```python
from build123d import *

# Parameters (mm, degrees)
F0_W     = 76.350024
F0_H     = 76.350024
F0_R     = 2.15265
F0_R_2   = 3
F0_R_3   = 15.497899
F1_DEPTH = 5.08
F2_R     = 4.7625


with BuildPart() as f1:
    # F0 (on Top) → F1 (new body)
    with BuildSketch(Plane.XY):
        Rectangle(F0_W, F0_H)
        with Locations((-33.412512, -33.412512)):
            Circle(F0_R, mode=Mode.SUBTRACT)
        with Locations((0, -32.000012)):
            Circle(F0_R_2, mode=Mode.SUBTRACT)
        with Locations((33.412512, -33.412512)):
            Circle(F0_R, mode=Mode.SUBTRACT)
        with Locations((-27.712823, 16.000006)):
            Circle(F0_R_2, mode=Mode.SUBTRACT)
        with Locations((-33.412512, 33.412512)):
            Circle(F0_R, mode=Mode.SUBTRACT)
        Circle(F0_R_3, mode=Mode.SUBTRACT)
        with Locations((27.712823, 16.000006)):
            Circle(F0_R_2, mode=Mode.SUBTRACT)
        with Locations((33.412512, 33.412512)):
            Circle(F0_R, mode=Mode.SUBTRACT)
    extrude(amount=F1_DEPTH)

    # F2
    f2_edges = [f1.edges().sort_by_distance(p)[0] for p in [
        (-38.175012, 38.175012, 2.54),
        (38.175012, 38.175012, 2.54),
        (38.175012, -38.175012, 2.54),
        (-38.175012, -38.175012, 2.54),
    ]]
    fillet(f2_edges, radius=F2_R)


solid = f1.part
```
Model file for the job. Use its own axes, mm. Give positions to 0.01 mm unless a question says otherwise; leave off trailing zeros. Loops run counter-clockwise (first coordinate to the right, second up) from the corner with the lowest first, then second, coordinate; pieces in that order, holes last. Notation, with made-up numbers: (87.5, -7) -> (140.5, -7) arc R23 cw to (140.5, 13) -> close; hole circle Ø11 at (86, 84). An arc over 180 degrees is marked (long way). Use CSV: the item, a comma, the result in double quotes. Start each with the question number.
1) Wall check: line 1 (X direction, y = 18, z = 0.9); line 2 (Y direction, x = -1.5, z = 1.2); line 3 (X direction, y = 18.5, z = 2.7). Give the ranges that are in metal, low to high.
2) Slice it at B-B on y = 0. Give the cut face in (x, z), plus the area to 3 significant figures.
3) Slice it at A-A on x = 0. Give the cut face in (y, z), plus the area to 3 significant figures.
4) Mould opens along Y. For faces 1 (the cylindrical face through (31.704, 32.103, 2.504)), 2 (the flat face through (38.175, 0, 3)), 3 (the cylindrical face through (36.74, 36.82, 2.58)), 4 (the cylindrical face through (-32.419, 31.503, 2.504)) say: released by +Y, released by -Y, zero draft, split by the parting line, or undercut.
5) Slice it at C-C on x = -8. Give the cut face in (y, z).
6) Slice it at D-D on z = 2.5. Give the number of separate pieces and of enclosed holes in the cut face, plus the area to 3 significant figures.
Computed values:
1,line 1,"x = -38.18 to -29.95, -25.48 to 25.48, 29.95 to 38.18"
1,line 2,"y = -38.18 to -34.6, -29.4 to -15.43, 15.43 to 38.18"
1,line 3,"x = -38.18 to -29.37, -26.05 to 26.05, 29.37 to 38.18"
2,outline,"(-38.18, 0) -> (-15.5, 0) -> (-15.5, 5.08) -> (-38.18, 5.08) -> close; (15.5, 0) -> (38.18, 0) -> (38.18, 5.08) -> (15.5, 5.08) -> close"
2,area,"230 mm^2"
3,outline,"(-38.18, 0) -> (-35, 0) -> (-35, 5.08) -> (-38.18, 5.08) -> close; (-29, 0) -> (-15.5, 0) -> (-15.5, 5.08) -> (-29, 5.08) -> close; (15.5, 0) -> (38.18, 0) -> (38.18, 5.08) -> (15.5, 5.08) -> close"
3,area,"200 mm^2"
4,face 1,"undercut"
4,face 2,"zero draft"
4,face 3,"released by +Y"
4,face 4,"undercut"
5,outline,"(-38.18, 0) -> (-13.27, 0) -> (-13.27, 5.08) -> (-38.18, 5.08) -> close; (13.27, 0) -> (38.18, 0) -> (38.18, 5.08) -> (13.27, 5.08) -> close"
6,separate pieces,"1"
6,enclosed holes,"8"
6,area,"4,910 mm^2"
